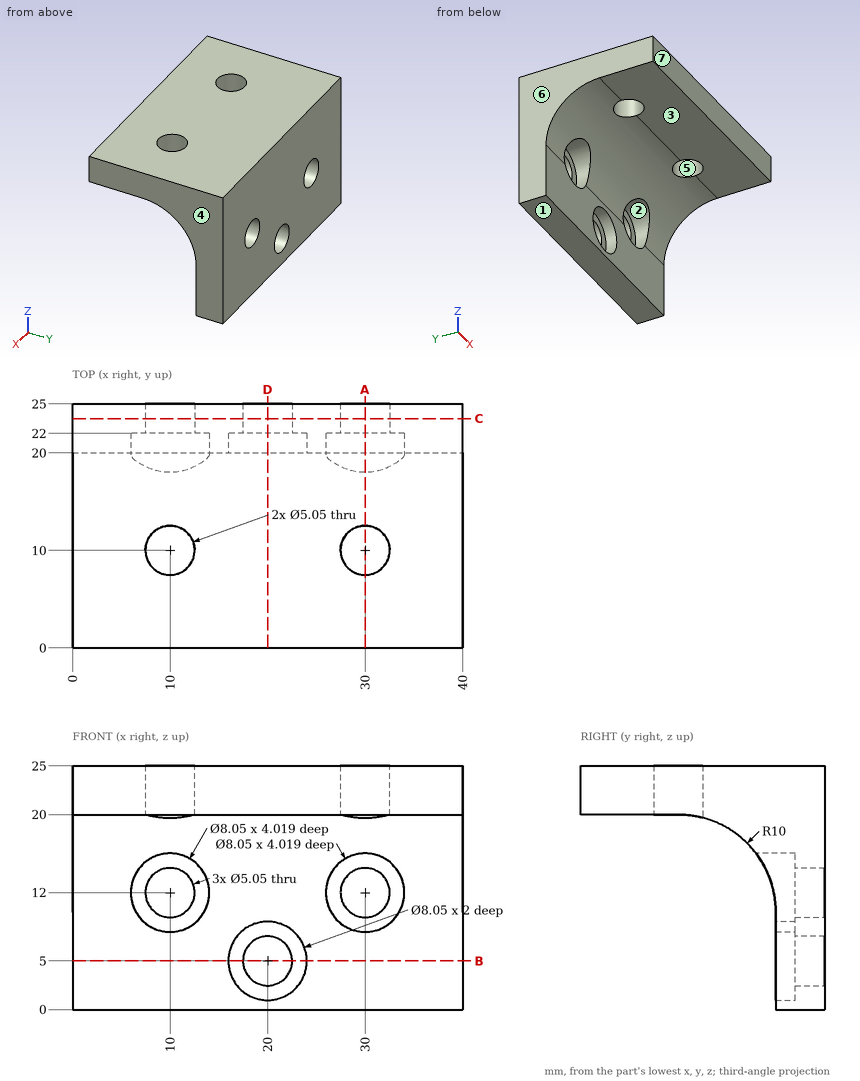
The drawing under review shows one solid part. Ordinate dimensions are in mm from its lowest x, y, z. A direction names the side the tool comes from. Round coordinates to 2 decimals unless told otherwise and drop trailing zeros. Loops run counter-clockwise (first coordinate to the right, second up) from the corner with the lowest first, then second, coordinate; pieces in that order, holes last. Notation, with made-up numbers: (-33.5, 79) - (-5.5, 79) arc R15 cw to (-5.5, 101) - close; hole circle Ø2 at (55, -32.75). An arc over 180 degrees is marked (long way). Use a Markdown table: item, result. Add a question column.
Q1. For probe 1 along X at (y, z) = (21.2, 12) (3 decimals); probe 2 along X at (y, z) = (10, 22.3) (3 decimals); probe 3 along Y at (x, z) = (10, 23.85) (3 decimals), list the stretches that pass through material, from the lowest coordinate up.
Q2. Add section C-C (y = 23.5). State the section outline as (x, z) points (3 decimals), plus the area to 3 significant figures.
Q3. Insertion check: pin 1 Ø2 at (x, y) = (17.5, 6.5) entering from -Z; pin 2 Ø6.5 at (x, z) = (21.5, 3.5) entering from -Y; pin 3 Ø6 at (x, z) = (20, 5) entering from -Y; pin 4 Ø6.5 at (x, z) = (30, 12) entering from +Y. Each pin has a flat end and moves straight along its axis. Give the tip position at first contact, or say it passes through.
Q4. Machinability: for the marked faces 1, 2 and 3, which of the approach directions +Z, -Z, +X, -X, +Y, -Y give a long, thin tool a straight path to every point of the face, cutting with its end or side? Answer none if there is none.
Q5. Add section B-B (z = 5). State the section outline as (x, y) points (3 decimals), plus the area to 3 significant figures.
Q6. Add section A-A (x = 30). State the section outline as (y, z) points (1 decimal).
Q7. Add section D-D (x = 20). State the section outline as (y, z) points (3 decimals), plus the area to 3 significant figures.
Q8. The part is to be moulded in two halves that separate along X. For the marked faces 4, 5, 6 and 7, say which applies: pulls with the +X half, pulls with the -X half, needs draft (parallel to the pull), parting line crosses it, or undercut.
Worked answers:
| question | item | result |
|---|---|---|
| 1 | probe 1 | 0 to 5.975, 14.025 to 25.975, 34.025 to 40 |
| 1 | probe 2 | 0 to 7.475, 12.525 to 27.475, 32.525 to 40 |
| 1 | probe 3 | 0 to 7.475, 12.525 to 25 |
| 2 | outline | (0, 0) - (40, 0) - (40, 25) - (0, 25) - close; hole circle Ø5.05 at (10, 12); hole circle Ø5.05 at (20, 5); hole circle Ø5.05 at (30, 12) |
| 2 | area | 940 mm² |
| 3 | pin 1 | z = 20 |
| 3 | pin 2 | y = 20 |
| 3 | pin 3 | y = 22 |
| 3 | pin 4 | y = 25 |
| 4 | face 1 | -Z, +X, -X, +Y, -Y |
| 4 | face 2 | -Y |
| 4 | face 3 | -Z, +X, -X, -Y |
| 5 | outline | (0, 20) - (15.975, 20) - (15.975, 22) - (17.475, 22) - (17.475, 25) - (0, 25) - close; (22.525, 22) - (24.025, 22) - (24.025, 20) - (40, 20) - (40, 25) - (22.525, 25) - close |
| 5 | area | 169 mm² |
| 6 | outline | (0, 20) - (7.5, 20) - (7.5, 25) - (0, 25) - close; (12.5, 19.7) arc R10 cw to (18, 16) - (22, 16) - (22, 14.5) - (25, 14.5) - (25, 25) - (12.5, 25) - close; (20, 0) - (25, 0) - (25, 9.5) - (22, 9.5) - (22, 8) - (20, 8) - close |
| 7 | outline | (0, 20) - (10, 20) arc R10 cw to (20, 10) - (20, 9.025) - (22, 9.025) - (22, 7.525) - (25, 7.525) - (25, 25) - (0, 25) - close; (20, 0) - (25, 0) - (25, 2.475) - (22, 2.475) - (22, 0.975) - (20, 0.975) - close |
| 7 | area | 215 mm² |
| 8 | face 4 | pulls with the +X half |
| 8 | face 5 | undercut |
| 8 | face 6 | pulls with the -X half |
| 8 | face 7 | needs draft |
